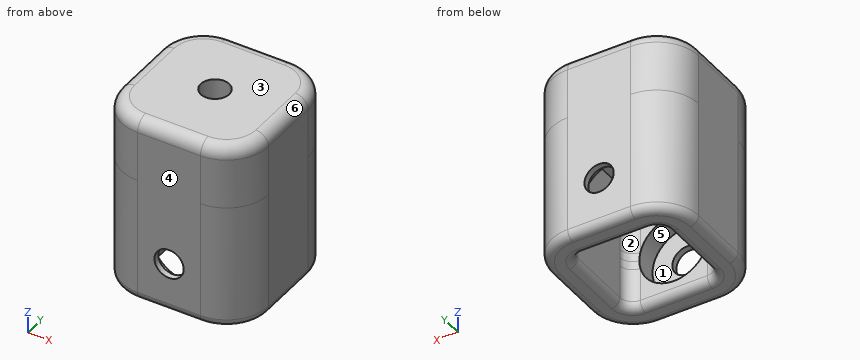
from build123d import *

# Parameters (mm, degrees)
SKETCH1_W                = 35
SKETCH1_H                = 35
SKETCH1_W_2              = 22
SKETCH1_H_2              = 22
BOSS_EXTRUDE1_DEPTH      = 30
SKETCH3_R                = 3.5
CUT_EXTRUDE2_DEPTH       = 36
SKETCH4_R                = 8.25
CUT_EXTRUDE3_DEPTH       = 5
FILLET1_R                = 10
FILLET4_R                = 2
FILLET5_R                = 3
NUT_RETENTION_AREA_DEPTH = 15
CUT_EXTRUDE5_DEPTH       = 8
SKETCH7_R                = 3.4
CUT_EXTRUDE6_DEPTH       = 46.0000001
FILLET6_R                = 3
FILLET7_R                = 2


with BuildPart() as part:
    # Sketch1 → Boss-Extrude1 (new body)
    with BuildSketch(Plane.XY):
        Rectangle(SKETCH1_W, SKETCH1_H)
        Rectangle(SKETCH1_W_2, SKETCH1_H_2, mode=Mode.SUBTRACT)
    extrude(amount=BOSS_EXTRUDE1_DEPTH)

    # Sketch3 → Cut-Extrude2 (cut, through all)
    with BuildSketch(Plane(origin=(0, 17.5, 0), x_dir=(1, 0, 0), z_dir=(0, 1, 0))):
        with Locations((0, -12)):
            Circle(SKETCH3_R)
    extrude(amount=-CUT_EXTRUDE2_DEPTH, mode=Mode.SUBTRACT)

    # Sketch4 → Cut-Extrude3 (cut)
    with BuildSketch(Plane(origin=(0, -11, 0), x_dir=(1, 0, 0), z_dir=(0, 1, 0))):
        with Locations((0, -12)):
            Circle(SKETCH4_R)
    cut_extrude3 = extrude(amount=-CUT_EXTRUDE3_DEPTH, mode=Mode.SUBTRACT)

    # Mirror2: Cut-Extrude3 across plane
    add(cut_extrude3.mirror(Plane.ZX), mode=Mode.SUBTRACT)

    # Fillet1
    fillet1_edges = [part.edges().sort_by_distance(p)[0] for p in [
        (17.5, -17.5, 15),
        (-17.5, -17.5, 15),
        (-17.5, 17.5, 15),
        (17.5, 17.5, 15),
    ]]
    fillet(fillet1_edges, radius=FILLET1_R)

    # Fillet4
    fillet4_edges = [part.edges().sort_by_distance(p)[0] for p in [
        (0, 17.5, 0),
        (17.5, 0, 0),
        (0, -17.5, 0),
        (-17.5, 0, 0),
        (-14.571067812, 14.571067812, 0),
        (-14.571067812, -14.571067812, 0),
        (14.571067812, -14.571067812, 0),
        (14.571067812, 14.571067812, 0),
    ]]
    fillet(fillet4_edges, radius=FILLET4_R)

    # Fillet5
    fillet5_edges = [part.edges().sort_by_distance(p)[0] for p in [
        (11, -11, 15),
        (11, 11, 15),
        (-11, 11, 15),
        (-11, -11, 15),
    ]]
    fillet(fillet5_edges, radius=FILLET5_R)

    # Sketch6 → Nut Retention Area (add)
    with BuildSketch(Plane.XY.offset(30)):
        with BuildLine():
            Line((7.5, 17.5), (-7.5, 17.5))
            ThreePointArc((-7.5, 17.5), (-14.571067812, 14.571067812), (-17.5, 7.5))
            Line((-17.5, 7.5), (-17.5, -7.5))
            ThreePointArc((-17.5, -7.5), (-14.571067812, -14.571067812), (-7.5, -17.5))
            Line((-7.5, -17.5), (7.5, -17.5))
            ThreePointArc((7.5, -17.5), (14.571067812, -14.571067812), (17.5, -7.5))
            Line((17.5, -7.5), (17.5, 7.5))
            ThreePointArc((17.5, 7.5), (14.571067812, 14.571067812), (7.5, 17.5))
        make_face()
    extrude(amount=NUT_RETENTION_AREA_DEPTH)

    # Sketch8 → Cut-Extrude5 (cut)
    with BuildSketch(Plane(origin=(0, 0, 30), x_dir=(-1, 0, 0), z_dir=(0, 0, -1))):
        Polygon((3.233161507, -5.6), (6.466323015, 0), (3.233161507, 5.6), (-3.233161507, 5.6), (-6.466323015, 0), (-3.233161507, -5.6), align=None)
    extrude(amount=-CUT_EXTRUDE5_DEPTH, mode=Mode.SUBTRACT)

    # Sketch7 → Cut-Extrude6 (cut, through all)
    with BuildSketch(Plane.XY.offset(45)):
        Circle(SKETCH7_R)
    extrude(amount=-CUT_EXTRUDE6_DEPTH, mode=Mode.SUBTRACT)

    # Fillet6
    fillet6_edges = [part.edges().sort_by_distance(p)[0] for p in [
        (-14.571067812, -14.571067812, 45),
        (0, -17.5, 45),
        (14.571067812, -14.571067812, 45),
        (17.5, 0, 45),
        (14.571067812, 14.571067812, 45),
        (0, 17.5, 45),
        (-14.571067812, 14.571067812, 45),
        (-17.5, 0, 45),
    ]]
    fillet(fillet6_edges, radius=FILLET6_R)

    # Fillet7
    fillet7_edges = [part.edges().sort_by_distance(p)[0] for p in [
        (0, 11, 0),
        (-11, 0, 0),
        (11, 0, 0),
        (0, -11, 0),
        (-10.121320344, 10.121320344, 0),
        (10.121320344, 10.121320344, 0),
        (10.121320344, -10.121320344, 0),
        (-10.121320344, -10.121320344, 0),
    ]]
    fillet(fillet7_edges, radius=FILLET7_R)


solid = part.part
Build history of the part. All positions in model axes, mm. Face numbers are marked on the shaded views. A direction names the side the tool comes from. Round coordinates to 2 decimals unless told otherwise and drop trailing zeros. Loops run counter-clockwise (first coordinate to the right, second up) from the corner with the lowest first, then second, coordinate; pieces in that order, holes last. Notation, with made-up numbers: (84.25, 9.25) -> (124.25, 9.25) arc R28 cw to (124.25, 30.25) -> close; hole circle Ø7 at (31, -17). An arc over 180 degrees is marked (long way). One line per item, written item: value. Start each with the question number.
Q1. Cut at A-A on z = 24. List the corners of the cut face in (x, y), plus the area to 3 significant figures.
Q2. Drop flat-ended pins along their axis: pin 1 Ø9 at (x, y) = (-1.5, 0) entering from -Z; pin 2 Ø5.5 at (x, z) = (0, 12) entering from +Y; pin 3 Ø3 at (x, z) = (13, 6) entering from -Y. Give the stop position or say it passes through.
Q3. Cut at C-C on x = 0. Count the separate pieces of the cut face and the enclosed holes in it, plus the area to 3 significant figures.
Q4. Probe line 1 along Y through (x, z) = (-6.5, 28); line 2 along Y through (x, z) = (-3, 31.5); line 3 along Z through (x, y) = (0, -13). List the from-to ranges inside material, lowest first.
Q5. Cut at B-B on y = -1. List the corners of the cut face in (x, z), plus the area to 3 significant figures.
Q6. Cut at D-D on z = 5. List the corners of the cut face in (x, y).
Q7. Two-plate mould, pull along Y, no slides. Class the marked faces 4, 5 and 6: released by +Y, released by -Y, zero draft, split by the parting line, or undercut.
Q8. 3-axis set-ups, long thin cutter, end or side, ignore diameter. For the marked faces 1, 2 and 3: which of +Z, -Z, +X, -X, +Y, -Y reach the whole face in a straight line?
Computed:
1. outline: (-17.5, -7.5) arc R10 ccw to (-7.5, -17.5) -> (7.5, -17.5) arc R10 ccw to (17.5, -7.5) -> (17.5, 7.5) arc R10 ccw to (7.5, 17.5) -> (-7.5, 17.5) arc R10 ccw to (-17.5, 7.5) -> close; hole (-11, -8) arc R3 ccw to (-8, -11) -> (8, -11) arc R3 ccw to (11, -8) -> (11, 8) arc R3 ccw to (8, 11) -> (-8, 11) arc R3 ccw to (-11, 8) -> close
1. area: 663 mm²
2. pin 1: z = 30
2. pin 2: through
2. pin 3: y = -16.67
3. separate pieces: 4
3. enclosed holes: 0
3. area: 585 mm²
4. line 1: -17.5 to -11, 11 to 17.5
4. line 2: -17.5 to -5.6, 5.6 to 17.5
4. line 3: 0 to 3.75, 20.25 to 45
5. outline: (-17.5, 2) arc R2 ccw to (-15.5, 0) -> (-13, 0) arc R2 ccw to (-11, 2) -> (-11, 30) -> (-5.89, 30) -> (-5.89, 38) -> (-3.25, 38) -> (-3.25, 45) -> (-14.5, 45) arc R3 ccw to (-17.5, 42) -> close; (3.25, 38) -> (5.89, 38) -> (5.89, 30) -> (11, 30) -> (11, 2) arc R2 ccw to (13, 0) -> (15.5, 0) arc R2 ccw to (17.5, 2) -> (17.5, 42) arc R3 ccw to (14.5, 45) -> (3.25, 45) -> close
5. area: 768 mm²
6. outline: (-17.5, -7.5) arc R10 ccw to (-7.5, -17.5) -> (7.5, -17.5) arc R10 ccw to (17.5, -7.5) -> (17.5, 7.5) arc R10 ccw to (7.5, 17.5) -> (-7.5, 17.5) arc R10 ccw to (-17.5, 7.5) -> close; hole (-11, -8) arc R3 ccw to (-8, -11) -> (-4.37, -11) -> (-4.37, -16) -> (4.37, -16) -> (4.37, -11) -> (8, -11) arc R3 ccw to (11, -8) -> (11, 8) arc R3 ccw to (8, 11) -> (4.37, 11) -> (4.37, 16) -> (-4.37, 16) -> (-4.37, 11) -> (-8, 11) arc R3 ccw to (-11, 8) -> close
7. face 4: released by -Y
7. face 5: undercut
7. face 6: zero draft
8. face 1: none
8. face 2: -Z
8. face 3: +Z, +X, -X, +Y, -Y
